from build123d import *

# Parameters (mm, degrees)
SKETCH1_W           = 106
SKETCH1_H           = 62
BOSS_EXTRUDE1_DEPTH = 2.5
FILLET1_R           = 1.5
BOSS_EXTRUDE2_DEPTH = 2
BOSS_EXTRUDE3_DEPTH = 1.25
SKETCH4_W           = 2.5
SKETCH4_H           = 9
SKETCH4_H_2         = 12.2
SKETCH4_H_3         = 48
BOSS_EXTRUDE4_DEPTH = 2


with BuildPart() as part:
    # Sketch1 → Boss-Extrude1 (new body)
    with BuildSketch(Plane(origin=(0, 0, 0), x_dir=(1, 0, 0), z_dir=(0, 1, 0))):
        with Locations((53, 31)):
            Rectangle(SKETCH1_W, SKETCH1_H)
    extrude(amount=BOSS_EXTRUDE1_DEPTH)

    # Fillet1
    fillet1_edges = [part.edges().sort_by_distance(p)[0] for p in [
        (0, 1.25, 0),
        (0, 1.25, -62),
        (106, 1.25, -62),
        (106, 1.25, 0),
    ]]
    fillet(fillet1_edges, radius=FILLET1_R)

    # Sketch2 → Boss-Extrude2 (add)
    with BuildSketch(Plane(origin=(0, 2.5, 0), x_dir=(1, 0, 0), z_dir=(0, 1, 0))):
        with BuildLine():
            Line((104.5, 62), (1.5, 62))
            ThreePointArc((1.5, 62), (0.439339828, 61.560660172), (0, 60.5))
            Line((0, 60.5), (0, 1.5))
            ThreePointArc((0, 1.5), (0.439339828, 0.439339828), (1.5, 0))
            Line((1.5, 0), (104.5, 0))
            ThreePointArc((104.5, 0), (105.560660172, 0.439339828), (106, 1.5))
            Line((106, 1.5), (106, 60.5))
            ThreePointArc((106, 60.5), (105.560660172, 61.560660172), (104.5, 62))
        make_face()
        with BuildLine():
            Line((102, 59.5), (4, 59.5))
            ThreePointArc((4, 59.5), (2.939339828, 59.060660172), (2.5, 58))
            Line((2.5, 58), (2.5, 4))
            ThreePointArc((2.5, 4), (2.939339828, 2.939339828), (4, 2.5))
            Line((4, 2.5), (102, 2.5))
            ThreePointArc((102, 2.5), (103.060660172, 2.939339828), (103.5, 4))
            Line((103.5, 4), (103.5, 58))
            ThreePointArc((103.5, 58), (103.060660172, 59.060660172), (102, 59.5))
        make_face(mode=Mode.SUBTRACT)
    extrude(amount=BOSS_EXTRUDE2_DEPTH)

    # Sketch3 → Boss-Extrude3 (add)
    with BuildSketch(Plane(origin=(0, 4.5, 0), x_dir=(1, 0, 0), z_dir=(0, 1, 0))):
        with BuildLine():
            Line((4, 1.5), (102, 1.5))
            ThreePointArc((102, 1.5), (103.767766953, 2.232233047), (104.5, 4))
            Line((104.5, 4), (104.5, 58))
            ThreePointArc((104.5, 58), (103.767766953, 59.767766953), (102, 60.5))
            Line((102, 60.5), (4, 60.5))
            ThreePointArc((4, 60.5), (2.232233047, 59.767766953), (1.5, 58))
            Line((1.5, 58), (1.5, 4))
            ThreePointArc((1.5, 4), (2.232233047, 2.232233047), (4, 1.5))
        make_face()
        with BuildLine():
            Line((4, 2.5), (102, 2.5))
            ThreePointArc((102, 2.5), (103.060660172, 2.939339828), (103.5, 4))
            Line((103.5, 4), (103.5, 58))
            ThreePointArc((103.5, 58), (103.060660172, 59.060660172), (102, 59.5))
            Line((102, 59.5), (4, 59.5))
            ThreePointArc((4, 59.5), (2.939339828, 59.060660172), (2.5, 58))
            Line((2.5, 58), (2.5, 4))
            ThreePointArc((2.5, 4), (2.939339828, 2.939339828), (4, 2.5))
        make_face(mode=Mode.SUBTRACT)
    extrude(amount=BOSS_EXTRUDE3_DEPTH)

    # Sketch4 → Boss-Extrude4 (add)
    with BuildSketch(Plane(origin=(0, 4.5, 0), x_dir=(1, 0, 0), z_dir=(0, 1, 0))):
        with Locations((1.25, 12.74)):
            Rectangle(SKETCH4_W, SKETCH4_H)
        with Locations((1.25, 42.79)):
            Rectangle(SKETCH4_W, SKETCH4_H_2)
        with Locations((104.75, 33.5)):
            Rectangle(SKETCH4_W, SKETCH4_H_3)
    extrude(amount=BOSS_EXTRUDE4_DEPTH)


solid = part.part
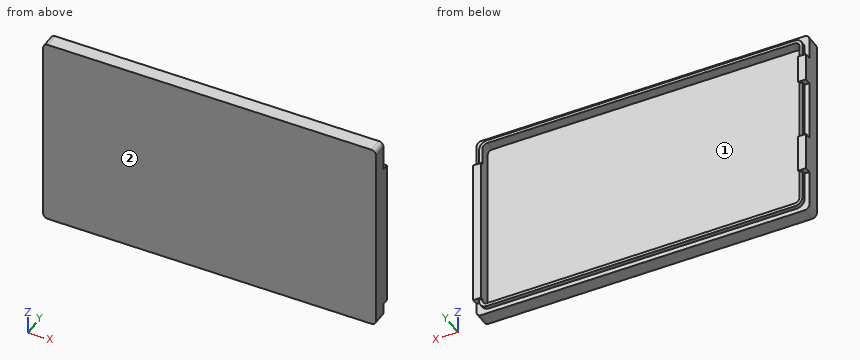
Geometry check sheet. Reference: the model listing, model coordinates, mm. Face numbers are marked on the shaded views. Coordinates: 2 decimals unless noted, no trailing zeros. Loops run counter-clockwise (first coordinate to the right, second up) from the corner with the lowest first, then second, coordinate; pieces in that order, holes last. Notation, with made-up numbers: (-39, 25) - (15, 25) arc R21 ccw to (15, 38) - close; hole circle Ø2 at (-8, -26.5). An arc over 180 degrees is marked (long way). Use one line per item in the form item = value. Start each with the question number.
Item 1: Section check A-A, the plane z = -56.5. Enter the section's corners in (x, y), and give its area (3 significant figures).
Item 2: Section check C-C, the plane z = -47.5. Enter the section's corners in (x, y).
Item 3: Section check B-B, the plane x = 83. Enter the section's corners in (y, z).
Item 4: Mould release check, pull along X, two halves, no side actions. Record for the marked faces 1 and 2: +X half, -X half, draft (parallel to the pull), parting line (faces both ways), or undercut.
Item 5: Gauge pin test, flat ends, axial feed: pin 1 (3 mm diameter, centred on y = 5.5, z = -9, fed in from +X); pin 2 (0.8 mm diameter, centred on x = 0.5, z = -22.5, fed in from +Y); pin 3 (5 mm diameter, centred on x = 49.5, z = -6.5, fed in from +Y); pin 4 (1 mm diameter, centred on y = 5.5, z = -30.5, fed in from -X). Record the tip position at first contact, or that the pin passes through.
Item 6: Thickness scan on probe 1 along X at (y, z) = (3, -5.5); probe 2 along Z at (x, y) = (101, 5.25); probe 3 along Z at (x, y) = (58, 3.25). Record the ranges inside material, lowest first.
Computed:
q1.outline = (0, 0) - (106, 0) - (106, 6.5) - (103.5, 6.5) - (103.5, 2.5) - (2.5, 2.5) - (2.5, 5.75) - (1.5, 5.75) - (1.5, 4.5) - (0, 4.5) - close
q1.area = 281 mm2
q2.outline = (0, 0) - (106, 0) - (106, 6.5) - (103.5, 6.5) - (103.5, 2.5) - (2.5, 2.5) - (2.5, 6.5) - (0, 6.5) - close
q3.outline = (0, -62) - (4.5, -62) - (4.5, -60.5) - (5.75, -60.5) - (5.75, -59.5) - (2.5, -59.5) - (2.5, -2.5) - (5.75, -2.5) - (5.75, -1.5) - (4.5, -1.5) - (4.5, 0) - (0, 0) - close
q4.face_1 = undercut
q4.face_2 = draft
q5.pin_1 = 106
q5.pin_2 = 4.5
q5.pin_3 = 2.5
q5.pin_4 = 1.5
q6.probe_1 = 0 to 2.5, 103.5 to 106
q6.probe_2 = -60.5 to -59.5, -2.5 to -1.5
q6.probe_3 = -62 to -59.5, -2.5 to 0
